from build123d import *

# Parameters (mm, degrees)
SKETCH1_R                                     = 4
BOSS_EXTRUDE1_DEPTH                           = 3.175
FILLET1_R                                     = 5.588
CSK_FOR_6_FLAT_HEAD_MACHINE_SCREW1_AT_2_COUNT = 2
CSK_FOR_6_FLAT_HEAD_MACHINE_SCREW1_AT_2_PITCH = 16
CSK_FOR_6_FLAT_HEAD_MACHINE_SCREW1_AT_3_COUNT = 2
CSK_FOR_6_FLAT_HEAD_MACHINE_SCREW1_AT_3_PITCH = 11.313708499
CSK_FOR_6_FLAT_HEAD_MACHINE_SCREW1_AT_4_COUNT = 2
CSK_FOR_6_FLAT_HEAD_MACHINE_SCREW1_AT_4_PITCH = 11.313708499
CSK_FOR_6_FLAT_HEAD_MACHINE_SCREW1_AT_5_COUNT = 2
CSK_FOR_6_FLAT_HEAD_MACHINE_SCREW1_AT_5_PITCH = 19.697715604
CSK_FOR_6_FLAT_HEAD_MACHINE_SCREW1_AT_6_COUNT = 2
CSK_FOR_6_FLAT_HEAD_MACHINE_SCREW1_AT_6_PITCH = 26
CSK_FOR_6_FLAT_HEAD_MACHINE_SCREW1_AT_7_COUNT = 2
CSK_FOR_6_FLAT_HEAD_MACHINE_SCREW1_AT_7_PITCH = 19.697715604
CSK_FOR_6_FLAT_HEAD_MACHINE_SCREW1_AT_8_COUNT = 2
CSK_FOR_6_FLAT_HEAD_MACHINE_SCREW1_AT_8_PITCH = 10
CSK_FOR_6_FLAT_HEAD_MACHINE_SCREW2_AT_2_COUNT = 2
CSK_FOR_6_FLAT_HEAD_MACHINE_SCREW2_AT_2_PITCH = 20
CSK_FOR_6_FLAT_HEAD_MACHINE_SCREW2_AT_3_COUNT = 2
CSK_FOR_6_FLAT_HEAD_MACHINE_SCREW2_AT_3_PITCH = 37.802116343
CSK_FOR_6_FLAT_HEAD_MACHINE_SCREW2_AT_4_COUNT = 2
CSK_FOR_6_FLAT_HEAD_MACHINE_SCREW2_AT_4_PITCH = 34.817380717
CSK_FOR_6_FLAT_HEAD_MACHINE_SCREW2_AT_5_COUNT = 2
CSK_FOR_6_FLAT_HEAD_MACHINE_SCREW2_AT_5_PITCH = 46
CSK_FOR_6_FLAT_HEAD_MACHINE_SCREW2_AT_6_COUNT = 2
CSK_FOR_6_FLAT_HEAD_MACHINE_SCREW2_AT_6_PITCH = 50.159744816
CSK_FOR_6_FLAT_HEAD_MACHINE_SCREW2_AT_7_COUNT = 2
CSK_FOR_6_FLAT_HEAD_MACHINE_SCREW2_AT_7_PITCH = 57.454329689
CSK_FOR_6_FLAT_HEAD_MACHINE_SCREW2_AT_8_COUNT = 2
CSK_FOR_6_FLAT_HEAD_MACHINE_SCREW2_AT_8_PITCH = 30.149626863
CSK_FOR_6_FLAT_HEAD_MACHINE_SCREW2_AT_9_COUNT = 2
CSK_FOR_6_FLAT_HEAD_MACHINE_SCREW2_AT_9_PITCH = 14.150971698


with BuildPart() as part:
    # Sketch1 → Boss-Extrude1 (new body)
    with BuildSketch(Plane.XY):
        with BuildLine():
            Line((-34, 71), (-34, -9.856977224))
            ThreePointArc((-34, -9.856977224), (0, -35.4), (34, -9.856977224))
            Line((34, -9.856977224), (34, 71))
            Line((34, 71), (-34, 71))
        make_face()
        Circle(SKETCH1_R, mode=Mode.SUBTRACT)
    extrude(amount=BOSS_EXTRUDE1_DEPTH)

    # Fillet1
    fillet1_edges = [part.edges().sort_by_distance(p)[0] for p in [
        (-34, 71, 1.5875),
        (34, 71, 1.5875),
    ]]
    fillet(fillet1_edges, radius=FILLET1_R)

    # Sketch7 → CSK for _6 Flat Head Machine Screw1 (revolve, cut)
    with BuildSketch(Plane(origin=(0, 8, 0), x_dir=(0, 1, 0), z_dir=(1, 0, 0))):
        Polygon((0, 0), (0, 3.175), (1.8288, 3.175), (1.8288, 1.972306634), (3.5433, 0), align=None)
    csk_for_6_flat_head_machine_screw1 = revolve(axis=Axis((0, 8, -6.35), (0, 0, 1)), mode=Mode.SUBTRACT)

    # CSK for _6 Flat Head Machine Screw1 at 2: CSK for _6 Flat Head Machine Screw1 ×2
    with Locations(*[(0, -i * CSK_FOR_6_FLAT_HEAD_MACHINE_SCREW1_AT_2_PITCH, 0) for i in range(1, CSK_FOR_6_FLAT_HEAD_MACHINE_SCREW1_AT_2_COUNT)]):
        add(csk_for_6_flat_head_machine_screw1, mode=Mode.SUBTRACT)

    # CSK for _6 Flat Head Machine Screw1 at 3: CSK for _6 Flat Head Machine Screw1 ×2
    with Locations(*[Vector(0.707106781, -0.707106781, 0) * (i * CSK_FOR_6_FLAT_HEAD_MACHINE_SCREW1_AT_3_PITCH) for i in range(1, CSK_FOR_6_FLAT_HEAD_MACHINE_SCREW1_AT_3_COUNT)]):
        add(csk_for_6_flat_head_machine_screw1, mode=Mode.SUBTRACT)

    # CSK for _6 Flat Head Machine Screw1 at 4: CSK for _6 Flat Head Machine Screw1 ×2
    with Locations(*[Vector(-0.707106781, -0.707106781, 0) * (i * CSK_FOR_6_FLAT_HEAD_MACHINE_SCREW1_AT_4_PITCH) for i in range(1, CSK_FOR_6_FLAT_HEAD_MACHINE_SCREW1_AT_4_COUNT)]):
        add(csk_for_6_flat_head_machine_screw1, mode=Mode.SUBTRACT)

    # CSK for _6 Flat Head Machine Screw1 at 5: CSK for _6 Flat Head Machine Screw1 ×2
    with Locations(*[Vector(0.913811549, -0.406138466, 0) * (i * CSK_FOR_6_FLAT_HEAD_MACHINE_SCREW1_AT_5_PITCH) for i in range(1, CSK_FOR_6_FLAT_HEAD_MACHINE_SCREW1_AT_5_COUNT)]):
        add(csk_for_6_flat_head_machine_screw1, mode=Mode.SUBTRACT)

    # CSK for _6 Flat Head Machine Screw1 at 6: CSK for _6 Flat Head Machine Screw1 ×2
    with Locations(*[(0, -i * CSK_FOR_6_FLAT_HEAD_MACHINE_SCREW1_AT_6_PITCH, 0) for i in range(1, CSK_FOR_6_FLAT_HEAD_MACHINE_SCREW1_AT_6_COUNT)]):
        add(csk_for_6_flat_head_machine_screw1, mode=Mode.SUBTRACT)

    # CSK for _6 Flat Head Machine Screw1 at 7: CSK for _6 Flat Head Machine Screw1 ×2
    with Locations(*[Vector(-0.913811549, -0.406138466, 0) * (i * CSK_FOR_6_FLAT_HEAD_MACHINE_SCREW1_AT_7_PITCH) for i in range(1, CSK_FOR_6_FLAT_HEAD_MACHINE_SCREW1_AT_7_COUNT)]):
        add(csk_for_6_flat_head_machine_screw1, mode=Mode.SUBTRACT)

    # CSK for _6 Flat Head Machine Screw1 at 8: CSK for _6 Flat Head Machine Screw1 ×2
    with Locations(*[(0, i * CSK_FOR_6_FLAT_HEAD_MACHINE_SCREW1_AT_8_PITCH, 0) for i in range(1, CSK_FOR_6_FLAT_HEAD_MACHINE_SCREW1_AT_8_COUNT)]):
        add(csk_for_6_flat_head_machine_screw1, mode=Mode.SUBTRACT)

    # Sketch9 → CSK for _6 Flat Head Machine Screw2 (revolve, cut)
    with BuildSketch(Plane(origin=(23, 36, 3.175), x_dir=(0, -1, 0), z_dir=(1, 0, 0))):
        Polygon((0, 0), (0, 3.175), (1.8288, 3.175), (1.8288, 1.972306634), (3.5433, 0), align=None)
    csk_for_6_flat_head_machine_screw2 = revolve(axis=Axis((23, 36, 9.525), (0, 0, -1)), mode=Mode.SUBTRACT)

    # CSK for _6 Flat Head Machine Screw2 at 2: CSK for _6 Flat Head Machine Screw2 ×2
    with Locations(*[(0, i * CSK_FOR_6_FLAT_HEAD_MACHINE_SCREW2_AT_2_PITCH, 0) for i in range(1, CSK_FOR_6_FLAT_HEAD_MACHINE_SCREW2_AT_2_COUNT)]):
        add(csk_for_6_flat_head_machine_screw2, mode=Mode.SUBTRACT)

    # CSK for _6 Flat Head Machine Screw2 at 3: CSK for _6 Flat Head Machine Screw2 ×2
    with Locations(*[Vector(-0.608431544, 0.793606361, 0) * (i * CSK_FOR_6_FLAT_HEAD_MACHINE_SCREW2_AT_3_PITCH) for i in range(1, CSK_FOR_6_FLAT_HEAD_MACHINE_SCREW2_AT_3_COUNT)]):
        add(csk_for_6_flat_head_machine_screw2, mode=Mode.SUBTRACT)

    # CSK for _6 Flat Head Machine Screw2 at 4: CSK for _6 Flat Head Machine Screw2 ×2
    with Locations(*[Vector(-0.976523773, 0.215409656, 0) * (i * CSK_FOR_6_FLAT_HEAD_MACHINE_SCREW2_AT_4_PITCH) for i in range(1, CSK_FOR_6_FLAT_HEAD_MACHINE_SCREW2_AT_4_COUNT)]):
        add(csk_for_6_flat_head_machine_screw2, mode=Mode.SUBTRACT)

    # CSK for _6 Flat Head Machine Screw2 at 5: CSK for _6 Flat Head Machine Screw2 ×2
    with Locations(*[(-i * CSK_FOR_6_FLAT_HEAD_MACHINE_SCREW2_AT_5_PITCH, 0, 0) for i in range(1, CSK_FOR_6_FLAT_HEAD_MACHINE_SCREW2_AT_5_COUNT)]):
        add(csk_for_6_flat_head_machine_screw2, mode=Mode.SUBTRACT)

    # CSK for _6 Flat Head Machine Screw2 at 6: CSK for _6 Flat Head Machine Screw2 ×2
    with Locations(*[Vector(-0.917070056, 0.398726111, 0) * (i * CSK_FOR_6_FLAT_HEAD_MACHINE_SCREW2_AT_6_PITCH) for i in range(1, CSK_FOR_6_FLAT_HEAD_MACHINE_SCREW2_AT_6_COUNT)]):
        add(csk_for_6_flat_head_machine_screw2, mode=Mode.SUBTRACT)

    # CSK for _6 Flat Head Machine Screw2 at 7: CSK for _6 Flat Head Machine Screw2 ×2
    with Locations(*[Vector(-0.852851304, 0.52215386, 0) * (i * CSK_FOR_6_FLAT_HEAD_MACHINE_SCREW2_AT_7_PITCH) for i in range(1, CSK_FOR_6_FLAT_HEAD_MACHINE_SCREW2_AT_7_COUNT)]):
        add(csk_for_6_flat_head_machine_screw2, mode=Mode.SUBTRACT)

    # CSK for _6 Flat Head Machine Screw2 at 8: CSK for _6 Flat Head Machine Screw2 ×2
    with Locations(*[Vector(0.099503719, 0.99503719, 0) * (i * CSK_FOR_6_FLAT_HEAD_MACHINE_SCREW2_AT_8_PITCH) for i in range(1, CSK_FOR_6_FLAT_HEAD_MACHINE_SCREW2_AT_8_COUNT)]):
        add(csk_for_6_flat_head_machine_screw2, mode=Mode.SUBTRACT)

    # CSK for _6 Flat Head Machine Screw2 at 9: CSK for _6 Flat Head Machine Screw2 ×2
    with Locations(*[Vector(-0.847998304, 0.52999894, 0) * (i * CSK_FOR_6_FLAT_HEAD_MACHINE_SCREW2_AT_9_PITCH) for i in range(1, CSK_FOR_6_FLAT_HEAD_MACHINE_SCREW2_AT_9_COUNT)]):
        add(csk_for_6_flat_head_machine_screw2, mode=Mode.SUBTRACT)


solid = part.part
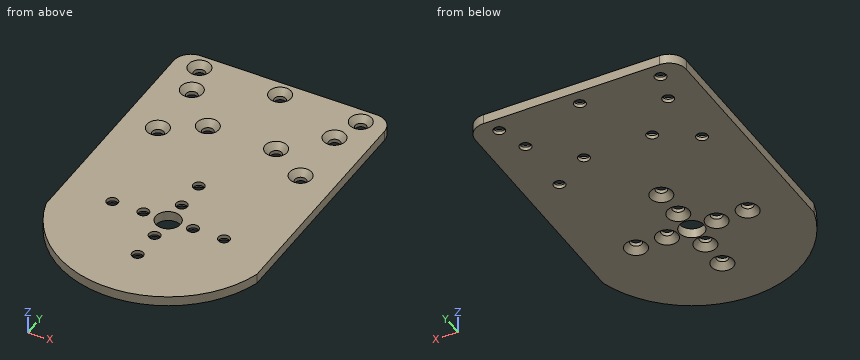
For this review, take the finished solid that the model builds, in its own axes (mm). Coordinates: 2 decimals unless noted, no trailing zeros. Order: outer loops, then holes, each group sorted by start corner. A loop starts at its lowest first (then second) coordinate and runs counter-clockwise, first axis right, second up. Notation, with made-up numbers: (81, 89.5) -> (140, 89.5) arc R22 cw to (140, 117.5) -> close; hole circle Ø8 at (39.25, -28). An arc over 180 degrees is marked (long way). Return JSON: item names as keys, results as strings.
1. For line 1 (X direction, y = 36, z = 0.85); line 2 (Y direction, x = -25, z = 2.55); line 3 (X direction, y = 18, z = 2.95), list the stretches that pass through material, from the lowest coordinate up. Write a range as from..to.
Answer block:
{"line 1": "-34..-24.83, -21.17..21.17, 24.83..34", "line 2": "-25.06..33.76, 38.24..53.76, 58.24..63.17, 68.83..71", "line 3": "-34..-1.83, 1.83..34"}
2. We need section D-D on y = -29. Write out the cut boundary in (x, z) (3 decimals), and give its area (3 significant figures).
Answer block:
{"outline": "(-20.302, 0) -> (20.302, 0) -> (20.302, 3.175) -> (-20.302, 3.175) -> close", "area": "129 mm²"}
3. We need section A-A on y = -8. Write out the cut boundary in (x, z) (3 decimals).
Answer block:
{"outline": "(-34, 0) -> (-3.543, 0) -> (-1.829, 1.972) -> (-1.829, 3.175) -> (-34, 3.175) -> close; (1.829, 1.972) -> (3.543, 0) -> (34, 0) -> (34, 3.175) -> (1.829, 3.175) -> close"}
4. We need section C-C on x = -18. Write out the cut boundary in (y, z) (3 decimals), and give its area (3 significant figures).
Answer block:
{"outline": "(-30.482, 0) -> (-3.543, 0) -> (-1.829, 1.972) -> (-1.829, 3.175) -> (-30.482, 3.175) -> close; (1.829, 1.972) -> (3.543, 0) -> (71, 0) -> (71, 3.175) -> (1.829, 3.175) -> close", "area": "307 mm²"}
5. We need section B-B on y = 56. Write out the cut boundary in (x, z) (3 decimals).
Answer block:
{"outline": "(-34, 0) -> (-24.829, 0) -> (-24.829, 1.203) -> (-26.543, 3.175) -> (-34, 3.175) -> close; (-21.171, 0) -> (21.171, 0) -> (21.171, 1.203) -> (19.457, 3.175) -> (-19.457, 3.175) -> (-21.171, 1.203) -> close; (24.829, 0) -> (34, 0) -> (34, 3.175) -> (26.543, 3.175) -> (24.829, 1.203) -> close"}
6. For pin 1 Ø2 at (x, y) = (-8, 0) entering from +Z; pin 2 Ø5 at (x, y) = (-23, 56) entering from +Z; pin 3 Ø6 at (x, y) = (23, 36) entering from +Z, all flat-tipped, find the tip position at first contact; note any pin that passes through.
Answer block:
{"pin 1": "through", "pin 2": "z = 1.97", "pin 3": "z = 2.55"}
